Here's how the part is built. I have some questions about the finished solid (model axes, mm). Round coordinates to 2 decimals unless told otherwise and drop trailing zeros. Loops run counter-clockwise (first coordinate to the right, second up) from the corner with the lowest first, then second, coordinate; pieces in that order, holes last. Notation, with made-up numbers: M 35,70 L 68,70 A28 cw 68,90 Z; hole C 22.5,32 d5. An arc over 180 degrees is marked long. Write each question's results on one line, items separated by ' | '. Start each with the question number.
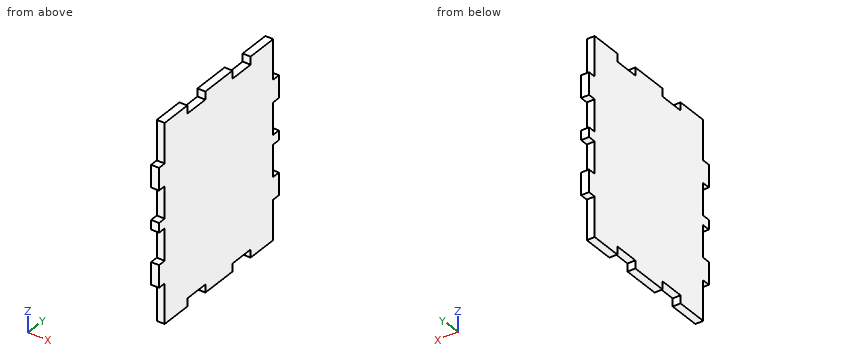
Autodesk Inventor part; units mm, degrees
ref_plane "YZ Plane" through (0, 0, 0) normal (1, 0, 0) x (0, 1, 0)
ref_plane "XZ Plane" through (0, 0, 0) normal (0, 1, 0) x (-1, 0, 0)
ref_plane "XY Plane" through (0, 0, 0) normal (0, 0, 1) x (1, 0, 0)
sketch "Sketch1" plane through (0, 0, 0) normal (1, 0, 0) x (0, 1, 0)
  line L0 (33.2271, 21.6336) -> (-27.7329, 21.6336)
  line L1 (-27.7329, 21.6336) -> (-27.7329, -50.7564)
  line L2 (-27.7329, -50.7564) -> (33.2271, -50.7564)
  line L3 (33.2271, -50.7564) -> (33.2271, 21.6336)
  line L4 (33.2271, -38.0564) -> (36.4021, -38.0564)
  line L5 (36.4021, -38.0564) -> (36.4021, -29.1664)
  line L6 (36.4021, -29.1664) -> (33.2271, -29.1664)
  line L7 (33.2271, -29.1664) -> (33.2271, -38.0564)
  line L8 (33.2271, 8.9336) -> (36.4021, 8.9336)
  line L9 (36.4021, 8.9336) -> (36.4021, 0.0436)
  line L10 (36.4021, 0.0436) -> (33.2271, 0.0436)
  line L11 (33.2271, 0.0436) -> (33.2271, 8.9336)
  line L12 (33.2271, -16.4664) -> (36.4021, -16.4664)
  line L13 (36.4021, -16.4664) -> (36.4021, -12.6564)
  line L14 (36.4021, -12.6564) -> (33.2271, -12.6564)
  line L15 (33.2271, -12.6564) -> (33.2271, -16.4664)
  line L16 (33.2271, 21.6336) -> (20.5271, 21.6336)
  line L17 (20.5271, 21.6336) -> (20.5271, 24.8086)
  line L18 (20.5271, 24.8086) -> (33.2271, 24.8086)
  line L19 (33.2271, 24.8086) -> (33.2271, 21.6336)
  line L20 (-27.7329, 21.6336) -> (-15.0329, 21.6336)
  line L21 (-15.0329, 21.6336) -> (-15.0329, 24.8086)
  line L22 (-15.0329, 24.8086) -> (-27.7329, 24.8086)
  line L23 (-27.7329, 24.8086) -> (-27.7329, 21.6336)
  line L24 (-4.8729, 21.6336) -> (10.3671, 21.6336)
  line L25 (10.3671, 21.6336) -> (10.3671, 24.8086)
  line L26 (10.3671, 24.8086) -> (-4.8729, 24.8086)
  line L27 (-4.8729, 24.8086) -> (-4.8729, 21.6336)
  point P0 (0, 0)
  dimension "d0" = 60.96
  dimension "d1" = 72.39
  dimension "d2" = 12.7
  dimension "d3" = 8.89
  dimension "d4" = 3.175
  dimension "d5" = 8.89
  dimension "d6" = 12.7
  dimension "d7" = 12.7
  dimension "d8" = 12.7
  dimension "d11" = 3.175
  dimension "d12" = 12.7
  dimension "d13" = 12.7
  dimension "d14" = 10.16
  dimension "d15" = 10.16
ref_plane "Work Plane1" through (0, 2.7471, 0.0436) normal (0, 1, 0) x (1, 0, 0)
extrude "Extrusion3" add sketch "Sketch1" along normal blind 3.175
ref_plane "Work Plane2" through (0, -15.0329, -14.5614) normal (0, 0, 1) x (1, 0, 0)
mirror "Mirror2" about plane through (0, -15.0329, -14.5614) normal (0, 0, 1) of "Extrusion3"
mirror "Mirror3" about plane through (0, 2.7471, 0.0436) normal (0, 1, 0) of "Extrusion3"
Item 1: I need wall thicknesses on L1, parallel to Z at x = 2.65, y = 33.5; L2, parallel to Z at x = 0.35, y = 14; L3, parallel to Y at x = 2.1, z = -28.5. Which ranges of each line are inside material? Lowest first, please.
Item 2: I'm going to push flat-ended pins straight in: pin 1 (1.6 mm diameter, centred on x = 2, z = -52.5, fed in from +Y); pin 2 (1.5 mm diameter, centred on x = 1.5, y = 14, fed in from +Z); pin 3 (1 mm diameter, centred on x = 1, z = 18, fed in from -Y). Where does each tip first touch, or does it pass through?
Item 3: If we section it at B-B on z = -7.5: Please give me the cut outline in (x, y) (3 decimals).
Item 4: If we section it at A-A on y = 13.5: Please give me the cut outline in (x, z) (3 decimals), and give its area (3 significant figures).
Numbers:
1) L1: -38.06 to -29.17, -16.47 to -12.66, 0.04 to 8.93 | L2: -50.76 to 21.63 | L3: -27.73 to 33.23
2) pin 1: y = 33.23 | pin 2: z = 21.63 | pin 3: y = -27.73
3) outline: M 0,-27.733 L 3.175,-27.733 L 3.175,33.227 L 0,33.227 Z
4) outline: M 0,-50.756 L 3.175,-50.756 L 3.175,21.634 L 0,21.634 Z | area: 230 mm²
